Here's how the part is built. I have some questions about the finished solid (model axes, mm). A direction names the side the tool comes from. Round coordinates to 2 decimals unless told otherwise and drop trailing zeros. Write each loop counter-clockwise with the first axis right and the second up, starting at its lowest first coordinate (ties: lowest second). Pieces come first, ordered by that corner, then holes. Notation, with made-up numbers: (27.25, 23.5) - (40.25, 23.5) arc R35 cw to (40.25, 58.5) - close; hole circle Ø10 at (57, -38.75). An arc over 180 degrees is marked (long way). Write item = value, one per line. Start each with the question number.
Item 1: Which directions (+Z, -Z, +X, -X, +Y, -Y) give clear straight access to the entire face, cutting with the end or side of a thin tool? Please do faces 1 (the face through (0.2, -14.7, 8.8)), 2 (the face through (-14.01, -19, 14)), 3 (the face through (7.8, 21.6, 8.9)), 4 (the face through (19, -21, 9)).
Item 2: If we section it at D-D (y = 12.5): Please give me the cut outline in (x, z), and give its area (3 significant figures).
Item 3: Thinking about a two-plate mould opening in Z: for faces 5 (the face through (-14.718, -15.421, 5.211)), 6 (the face through (0, -21, 9)), 7 (the face through (16, 18, 9.52)), which applies, pulls with the +Z half, pulls with the -Z half, needs draft (parallel to the pull), parting line crosses it, or undercut?
Item 4: For P1, Ø1, axis at x = -5, z = 7.5, coming from the -Y side; P2, Ø4, axis at x = 12.5, y = -12.5, coming from the -Z side; P3, Ø2, axis at x = -5, y = -10.5, coming from the -Z side; P4, Ø3, axis at y = 19, z = 14.5, coming from the +X side, each with a flat end and sliding along its axis, tell me the tip position at first contact or that it passes through.
Item 5: If we section it at A-A (x = 0): Please give me the cut outline in (y, z) (3 decimals), and give its area (3 significant figures).
Item 6: If I drill on line 1 along Y through (x, z) = (-12, 11.25); line 2 along X through (y, z) = (-19, 0.75); line 3 along Y through (x, z) = (2.5, 11), over which ranges is the centre line in solid material (lowest first)? Write a range as [from, to].
Item 7: If we section it at C-C (x = -17.51): Please give me the cut outline in (y, z) (3 decimals), and give its area (3 significant figures).
Item 8: If we section it at B-B (y = 8): Please give me the cut outline in (x, z), and give its area (3 significant figures).
```python
from build123d import *

# Parameters (mm, degrees)
BOSS_EXTRUDE2_DEPTH     = 18
SKETCH2_R               = 19.825
CUT_EXTRUDE1_DEPTH      = 2.5
SKETCH3_R               = 14.7
CUT_EXTRUDE2_DEPTH      = 14.5
CUT_EXTRUDE3_DEPTH      = 14.5
SKETCH5_R               = 10.5
CUT_EXTRUDE4_DEPTH      = 14.5
SKETCH7_R               = 2.5
SKETCH7_R_2             = 2.02
CUT_EXTRUDE6_DEPTH      = 30
CUT_EXTRUDE6_DEPTH_BACK = 60
SKETCH9_R               = 1.623885446
SKETCH9_R_2             = 2.25
CUT_EXTRUDE7_DEPTH      = 30
CUT_EXTRUDE8_DEPTH      = 8.48


with BuildPart() as part:
    # Sketch1 → Boss-Extrude2 (new body)
    with BuildSketch(Plane.XY):
        Polygon((-7.2, 21), (7.2, 21), (8.43, 22.23), (16.98, 22.23), (18.21, 21), (20.01, 21), (21.01, 20), (21.01, -20), (20.01, -21), (18.21, -21), (16.98, -22.23), (8.43, -22.23), (7.2, -21), (-7.2, -21), (-8.43, -22.23), (-16.98, -22.23), (-18.21, -21), (-20.01, -21), (-21.01, -20), (-21.01, 20), (-20.01, 21), (-18.21, 21), (-16.98, 22.23), (-8.43, 22.23), align=None)
    extrude(amount=BOSS_EXTRUDE2_DEPTH)

    # Sketch2 → Cut-Extrude1 (cut)
    with BuildSketch(Plane.XY.offset(18)):
        Circle(SKETCH2_R)
    extrude(amount=-CUT_EXTRUDE1_DEPTH, mode=Mode.SUBTRACT)

    # Sketch3 → Cut-Extrude2 (cut)
    with BuildSketch(Plane(origin=(0, 0, 0), x_dir=(-1, 0, 0), z_dir=(0, 0, -1))):
        Circle(SKETCH3_R)
    extrude(amount=-CUT_EXTRUDE2_DEPTH, mode=Mode.SUBTRACT)

    # Sketch4 → Cut-Extrude3 (cut)
    with BuildSketch(Plane(origin=(0, 0, 0), x_dir=(-1, 0, 0), z_dir=(0, 0, -1))):
        Polygon((18.8, 0), (18.8, 8.8), (-18.8, 8.8), (-18.8, -8.8), (18.8, -8.8), align=None)
    extrude(amount=-CUT_EXTRUDE3_DEPTH, mode=Mode.SUBTRACT)

    # Sketch5 → Cut-Extrude4 (cut)
    with BuildSketch(Plane(origin=(0, 0, 14.5), x_dir=(-1, 0, 0), z_dir=(0, 0, -1))):
        Circle(SKETCH5_R)
    extrude(amount=-CUT_EXTRUDE4_DEPTH, mode=Mode.SUBTRACT)

    # Sketch7 → Cut-Extrude6 (cut, two sides)
    with BuildSketch(Plane(origin=(0, 21, 0), x_dir=(1, 0, 0), z_dir=(0, 1, 0))) as cut_extrude6_sk:
        with Locations((0, -5.3)):
            Circle(SKETCH7_R)
        with Locations((12.7, -5.3)):
            Circle(SKETCH7_R_2)
        with Locations((-12.7, -5.3)):
            Circle(SKETCH7_R_2)
    extrude(amount=CUT_EXTRUDE6_DEPTH, mode=Mode.SUBTRACT)
    extrude(cut_extrude6_sk.sketch, amount=-CUT_EXTRUDE6_DEPTH_BACK, mode=Mode.SUBTRACT)

    # Sketch9 → Cut-Extrude7 (cut)
    with BuildSketch(Plane.XY.offset(18)):
        with Locations((17.97, 17.97)):
            Circle(SKETCH9_R)
        with Locations((-17.51, 17.505)):
            Circle(SKETCH9_R_2)
        with Locations((17.51, -17.505)):
            Circle(SKETCH9_R_2)
        with Locations((-17.97, -17.97)):
            Circle(SKETCH9_R)
    extrude(amount=-CUT_EXTRUDE7_DEPTH, mode=Mode.SUBTRACT)

    # Sketch10 → Cut-Extrude8 (cut)
    with BuildSketch(Plane.XY.offset(18)):
        Polygon((14.01, 22.23), (14.01, 16), (16.01, 14), (21.01, 14), (21.01, 20), (20.01, 21), (18.21, 21), (16.98, 22.23), align=None)
        Polygon((-21.01, -14), (-16.01, -14), (-14.01, -16), (-14.01, -22.23), (-16.98, -22.23), (-18.21, -21), (-20.01, -21), (-21.01, -20), align=None)
    extrude(amount=-CUT_EXTRUDE8_DEPTH, mode=Mode.SUBTRACT)


solid = part.part
```
Reply:
q1.face_1 = -Z
q1.face_2 = +Z, -X, -Y
q1.face_3 = +Z, -Z, +Y
q1.face_4 = +Z, -Z, +X, -Y
q2.outline = (-21.01, 0) - (-7.74, 0) - (-7.74, 14.5) - (7.74, 14.5) - (7.74, 0) - (21.01, 0) - (21.01, 18) - (15.39, 18) - (15.39, 15.5) - (-15.39, 15.5) - (-15.39, 18) - (-21.01, 18) - close; hole circle Ø4.04 at (-12.7, 5.3); hole circle Ø4.04 at (12.7, 5.3)
q2.area = 429 mm2
q3.face_5 = undercut
q3.face_6 = needs draft
q3.face_7 = pulls with the +Z half
q4.P1 = -21
q4.P2 = 0
q4.P3 = 14.5
q4.P4 = 14.01
q5.outline = (-21, 0) - (-14.7, 0) - (-14.7, 2.8) - (-21, 2.8) - close; (-21, 7.8) - (-14.7, 7.8) - (-14.7, 14.5) - (-10.5, 14.5) - (-10.5, 15.5) - (-19.825, 15.5) - (-19.825, 18) - (-21, 18) - close; (10.5, 14.5) - (14.7, 14.5) - (14.7, 7.8) - (21, 7.8) - (21, 18) - (19.825, 18) - (19.825, 15.5) - (10.5, 15.5) - close; (14.7, 0) - (21, 0) - (21, 2.8) - (14.7, 2.8) - close
q5.area = 147 mm2
q6.line_1 = [-22.23, -8.8], [8.8, 22.23]
q6.line_2 = [-21.01, -19.23], [-16.71, 15.83], [19.19, 21.01]
q6.line_3 = [-21, -14.49], [14.49, 21]
q7.outline = (-21.7, 0) - (-19.527, 0) - (-19.527, 9.52) - (-21.7, 9.52) - close; (-16.413, 0) - (-8.8, 0) - (-8.8, 14.5) - (8.8, 14.5) - (8.8, 0) - (15.255, 0) - (15.255, 18) - (9.297, 18) - (9.297, 15.5) - (-9.297, 15.5) - (-9.297, 18) - (-14, 18) - (-14, 9.52) - (-16.413, 9.52) - close; (19.755, 0) - (21.7, 0) - (21.7, 18) - (19.755, 18) - close
q7.area = 304 mm2
q8.outline = (-21.01, 0) - (-18.8, 0) - (-18.8, 14.5) - (-6.8, 14.5) - (-6.8, 15.5) - (-18.14, 15.5) - (-18.14, 18) - (-21.01, 18) - close; (6.8, 14.5) - (18.8, 14.5) - (18.8, 0) - (21.01, 0) - (21.01, 18) - (18.14, 18) - (18.14, 15.5) - (6.8, 15.5) - close
q8.area = 107 mm2
